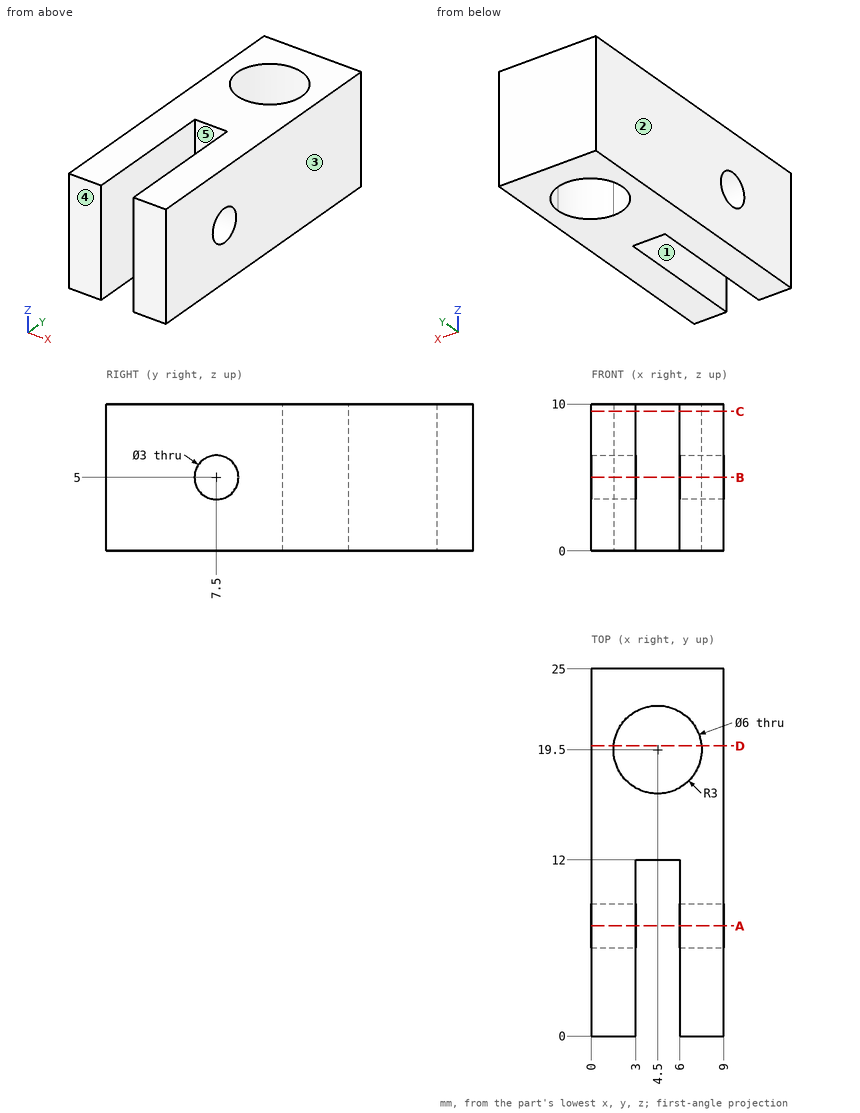
Could you check a few things on this drawing? It's one solid part, dimensions in mm from its lowest x, y, z. A direction names the side the tool comes from. Round coordinates to 2 decimals unless told otherwise and drop trailing zeros. Write each loop counter-clockwise with the first axis right and the second up, starting at its lowest first coordinate (ties: lowest second). Pieces come first, ordered by that corner, then holes. Notation, with made-up numbers: (-12.75, 78.25) -> (7.25, 78.25) arc R12 ccw to (7.25, 101.25) -> close; hole circle Ø7 at (21.5, 85.25). An arc over 180 degrees is marked (long way). One line per question, with ' | ' between items. Start each with the question number.
1) Suppose I cut it at A-A on y = 7.5. Write out the boundary of the cut face in (x, z), then the cut area to 3 significant figures.
2) Suppose I cut it at D-D on y = 19.75. Write out the boundary of the cut face in (x, z), then the cut area to 3 significant figures.
3) On a 3-axis mill with a long thin cutter (end or side, diameter ignored), from which of +Z, -Z, +X, -X, +Y, -Y can I reach the whole of each face in a straight line? I mean the marked faces 1 and 2. Say none if no direction works.
4) Suppose I cut it at C-C on z = 9.5. Write out the boundary of the cut face in (x, y).
5) If we mould it in two halves opening along X, with no side actions, what happens to the marked faces 3, 4 and 5? For each: released by +X, released by -X, zero draft, split by the parting line, or undercut.
6) I need wall thicknesses on line 1 (Y direction, x = 4.5, z = 5.25); line 2 (X direction, y = 5.25, z = 7); line 3 (Y direction, x = 8.35, z = 5). Which ranges of each line are inside material? Lowest first, please. Write a range as [from, to].
7) Suppose I cut it at B-B on z = 5. Write out the boundary of the cut face in (x, y).
Return value:
1) outline: (0, 0) -> (3, 0) -> (3, 3.5) -> (0, 3.5) -> close; (0, 6.5) -> (3, 6.5) -> (3, 10) -> (0, 10) -> close; (6, 0) -> (9, 0) -> (9, 3.5) -> (6, 3.5) -> close; (6, 6.5) -> (9, 6.5) -> (9, 10) -> (6, 10) -> close | area: 42.0 mm2
2) outline: (0, 0) -> (1.51, 0) -> (1.51, 10) -> (0, 10) -> close; (7.49, 0) -> (9, 0) -> (9, 10) -> (7.49, 10) -> close | area: 30.2 mm2
3) face 1: +Z, -Z, -Y | face 2: +Z, -Z, -X, +Y, -Y
4) outline: (0, 0) -> (3, 0) -> (3, 12) -> (6, 12) -> (6, 0) -> (9, 0) -> (9, 25) -> (0, 25) -> close; hole circle Ø6 at (4.5, 19.5)
5) face 3: released by +X | face 4: zero draft | face 5: undercut
6) line 1: y = [12, 16.5], [22.5, 25] | line 2: x = [0, 3], [6, 9] | line 3: y = [0, 6], [9, 25]
7) outline: (0, 0) -> (3, 0) -> (3, 6) -> (0, 6) -> close; (0, 9) -> (3, 9) -> (3, 12) -> (6, 12) -> (6, 9) -> (9, 9) -> (9, 25) -> (0, 25) -> close; (6, 0) -> (9, 0) -> (9, 6) -> (6, 6) -> close; hole circle Ø6 at (4.5, 19.5)
